```python
from build123d import *

# Parameters (mm, degrees)
BOSS_EXTRUDE1_DEPTH = 20
SHELL4_T            = 2
FILLET2_R           = 5
SKETCH3_W           = 21.5
SKETCH3_H           = 30
BOSS_EXTRUDE2_DEPTH = 20
SKETCH4_W           = 17.5
SKETCH4_H           = 28
CUT_EXTRUDE1_DEPTH  = 3.3
CUT_EXTRUDE2_DEPTH  = 2


with BuildPart() as part:
    # Sketch2 → Boss-Extrude1 (new body)
    with BuildSketch(Plane(origin=(0, 0, 0), x_dir=(0, 0, -1), z_dir=(1, 0, 0))):
        with BuildLine():
            Line((-27.001202387, 32.141013477), (-22.602835252, -36.63027149))
            ThreePointArc((-22.602835252, -36.63027149), (-19.464913087, -43.285247796), (-12.623224858, -45.992011054))
            Line((-12.623224858, -45.992011054), (12.623224858, -45.992011054))
            ThreePointArc((12.623224858, -45.992011054), (19.464913087, -43.285247796), (22.602835252, -36.63027149))
            Line((22.602835252, -36.63027149), (27.001202387, 32.141013477))
            ThreePointArc((27.001202387, 32.141013477), (25.118351891, 38.648045435), (19.520174304, 42.462098214))
            ThreePointArc((19.520174304, 42.462098214), (0, 44.940033366), (-19.520174304, 42.462098214))
            ThreePointArc((-19.520174304, 42.462098214), (-25.118351891, 38.648045435), (-27.001202387, 32.141013477))
        make_face()
    extrude(amount=BOSS_EXTRUDE1_DEPTH)

    # Shell4
    shell4_openings = [part.faces().sort_by_distance(p)[0] for p in [
        (20, 0.52350314, 0),
    ]]
    offset(amount=SHELL4_T, openings=shell4_openings, kind=Kind.INTERSECTION)

    # Fillet2
    # the kernel refuses this fillet: 5 mm, written as the material it takes off along each edge
    with BuildSketch(Plane(origin=(-2, -47.992011054, 12.623224858), x_dir=(1, 0, 0), z_dir=(0, 0, -1))) as fillet2_piece_1:
        with BuildLine():
            CenterArc((FILLET2_R, -FILLET2_R), FILLET2_R, 90, 90)
            Line((0, -FILLET2_R), (0, 0))
            Line((0, 0), (FILLET2_R, 0))
        make_face()
    extrude(amount=25.246449717, mode=Mode.SUBTRACT)
    with BuildSketch(Plane(origin=(-2, -35.992011054, 12.623224858), x_dir=(0, -1, 0), z_dir=(0, 0, -1))) as fillet2_piece_2:
        with BuildLine():
            CenterArc((12 - FILLET2_R, -FILLET2_R), FILLET2_R, 0, 90)
            Line((12 - FILLET2_R, 0), (12, 0))
            Line((12, 0), (12, -FILLET2_R))
        make_face()
    revolve(axis=Axis((-2, -35.992011054, 12.623224858), (-1, 0, 0)), revolution_arc=86.340549578, mode=Mode.SUBTRACT)
    with BuildSketch(Plane(origin=(-2, 32.01336139, 28.997124466), x_dir=(1, 0, 0), z_dir=(0, -0.997961039394411, -0.06382604367205215)), Plane(origin=(-2, -36.757923578, -24.598757331), x_dir=(1, 0, 0), z_dir=(0, 0.9979610393944109, -0.06382604367205376))) as fillet2_piece_3:
        with BuildLine():
            CenterArc((FILLET2_R, -FILLET2_R), FILLET2_R, 90, 90)
            Line((0, -FILLET2_R), (0, 0))
            Line((0, 0), (FILLET2_R, 0))
        make_face()
    extrude(amount=68.911793399, mode=Mode.SUBTRACT)
    with BuildSketch(Plane(origin=(-2, 32.779273914, 17.021591993), x_dir=(0, -0.06382604367205197, 0.997961039394411), z_dir=(0, -0.997961039394411, -0.06382604367205197))) as fillet2_piece_4:
        with BuildLine():
            CenterArc((12 - FILLET2_R, -FILLET2_R), FILLET2_R, 0, 90)
            Line((12 - FILLET2_R, 0), (12, 0))
            Line((12, 0), (12, -FILLET2_R))
        make_face()
    revolve(axis=Axis((-2, 32.779273914, 17.021591993), (-1, 0, 0)), revolution_arc=79.190327228, mode=Mode.SUBTRACT)
    with BuildSketch(Plane(origin=(-2, -33.184966634, 0), x_dir=(0, 0.9682824300555203, 0.249858231094708), z_dir=(0, -0.249858231094708, 0.9682824300555203))) as fillet2_piece_5:
        with BuildLine():
            CenterArc((80.125 - FILLET2_R, -FILLET2_R), FILLET2_R, 0, 90)
            Line((80.125 - FILLET2_R, 0), (80.125, 0))
            Line((80.125, 0), (80.125, -FILLET2_R))
        make_face()
    revolve(axis=Axis((-2, -33.184966634, 0), (-1, 0, 0)), revolution_arc=28.938246388, mode=Mode.SUBTRACT)
    with BuildSketch(Plane(origin=(-2, 32.779273914, -17.021591993), x_dir=(0, 0.9682824300555204, -0.24985823109470737), z_dir=(0, 0.24985823109470737, 0.9682824300555204))) as fillet2_piece_6:
        with BuildLine():
            CenterArc((12 - FILLET2_R, -FILLET2_R), FILLET2_R, 0, 90)
            Line((12 - FILLET2_R, 0), (12, 0))
            Line((12, 0), (12, -FILLET2_R))
        make_face()
    revolve(axis=Axis((-2, 32.779273914, -17.021591993), (-1, 0, 0)), revolution_arc=79.190327228, mode=Mode.SUBTRACT)
    with BuildSketch(Plane(origin=(-2, -35.992011054, -12.623224858), x_dir=(0, -0.06382604367205372, -0.9979610393944109), z_dir=(0, 0.9979610393944109, -0.06382604367205372))) as fillet2_piece_7:
        with BuildLine():
            CenterArc((12 - FILLET2_R, -FILLET2_R), FILLET2_R, 0, 90)
            Line((12 - FILLET2_R, 0), (12, 0))
            Line((12, 0), (12, -FILLET2_R))
        make_face()
    revolve(axis=Axis((-2, -35.992011054, -12.623224858), (-1, 0, 0)), revolution_arc=86.340549578, mode=Mode.SUBTRACT)

    # Sketch3 → Boss-Extrude2 (add)
    with BuildSketch(Plane(origin=(0, 0, 0), x_dir=(0, 0, -1), z_dir=(1, 0, 0))):
        with Locations((0, -30.992011054)):
            Rectangle(SKETCH3_W, SKETCH3_H)
    extrude(amount=BOSS_EXTRUDE2_DEPTH)

    # Sketch4 → Cut-Extrude1 (cut)
    with BuildSketch(Plane(origin=(20, 0, 0), x_dir=(0, 0, -1), z_dir=(1, 0, 0))):
        with Locations((0, -31.992011054)):
            Rectangle(SKETCH4_W, SKETCH4_H)
    extrude(amount=-CUT_EXTRUDE1_DEPTH, mode=Mode.SUBTRACT)

    # Sketch5 → Cut-Extrude2 (cut)
    with BuildSketch(Plane.XZ.offset(47.992011054)):
        with BuildLine():
            Line((20, 2.351775142), (20, -6.648224858))
            ThreePointArc((20, -6.648224858), (18.961461825, -6.347856856), (18.3, -5.492724858))
            Line((18.3, -5.492724858), (18.3, 1.197275142))
            ThreePointArc((18.3, 1.197275142), (18.954546218, 2.062330624), (20, 2.351775142))
        make_face()
    extrude(amount=-CUT_EXTRUDE2_DEPTH, mode=Mode.SUBTRACT)


solid = part.part
```
Source: CAD feature listing. Evaluate the final solid. Frame: model axes, mm. A direction names the side the tool comes from. Coordinates: 2 decimals unless noted, no trailing zeros. Write each loop counter-clockwise with the first axis right and the second up, starting at its lowest first coordinate (ties: lowest second). Pieces come first, ordered by that corner, then holes. Notation, with made-up numbers: M -10.5,-11 L 28.5,-11 A10 ccw 28.5,-3 Z; hole C 89,12 d4. An arc over 180 degrees is marked long. Answer as a JSON object with one key per item and string values.
1. Access query for faces 1 (the cylindrical face through (-0.496, -46.566, 0.177)), 2 (the flat face through (18.3, -47, -2)), 3 (the flat face through (18, -32, -8.75)). Directions: +Z, -Z, +X, -X, +Y, -Y. A direction counts if a zero-diameter tool reaches every point of the face in a straight line with its end or side. Return the directions, or none.
Evaluation:
{"face 1": "+Z, -Z, -X, -Y", "face 2": "+X, -Y", "face 3": "+X"}
2. Draft query along Y for faces 4 (the flat face through (-2, 0, 0)), 5 (the flat face through (11.38, -1.89, 26.83)), 6 (the cylindrical face through (9.86, -43.213, 19.541)). Return one class per face: released by +Y, released by -Y, zero draft, split by the parting line, or undercut.
Evaluation:
{"face 4": "zero draft", "face 5": "released by -Y", "face 6": "undercut"}
3. Contact query for flat-ended pins moving along their axis: P1, Ø1.5, axis at x = 14, y = 28.5, coming from the +Z side; P2, Ø6, axis at x = 10, y = -25.5, coming from the +Z side; P3, Ø1, axis at x = 19, y = -32, coming from the +Z side. Output: stop coordinate, or through.
Evaluation:
{"P1": "z = 28.82", "P2": "z = 25.51", "P3": "z = 24.94"}
4. Cut plane A-A on x = 7.5. Output: boundary loops of the cut face in (y, z) (3 decimals), plus the area to 3 significant figures.
Evaluation:
{"outline": "M -47.992,-12.623 A12 ccw -36.758,-24.599 L 32.013,-28.997 A12 ccw 44.399,-20.02 A80.125 ccw 44.399,20.02 A12 ccw 32.013,28.997 L -36.758,24.599 A12 ccw -47.992,12.623 Z; hole M -45.992,-12.623 A10 ccw -36.63,-22.603 L 32.141,-27.001 A10 ccw 42.462,-19.52 A78.125 ccw 42.462,19.52 A10 ccw 32.141,27.001 L -36.63,22.603 A10 ccw -45.992,12.623 L -45.992,10.75 L -15.992,10.75 L -15.992,-10.75 L -45.992,-10.75 Z", "area": "1,180 mm^2"}
5. Ray query, L1, parallel to Y at x = 18.25, z = 5; L2, parallel to Z at x = 4.75, y = -19.5; L3, parallel to X at y = 30, z = -6. Return the intervals inside material, ascending.
Evaluation:
{"L1": "-47.99 to -45.99, -17.99 to -15.99, 44.78 to 46.78", "L2": "-25.7 to -23.7, -10.75 to 10.75, 23.7 to 25.7", "L3": "-2 to 0"}
6. Cut plane B-B on x = 2. Output: boundary loops of the cut face in (y, z) (3 decimals), plus the area to 3 significant figures.
Evaluation:
{"outline": "M -47.891,-12.623 A11.899 ccw -36.751,-24.498 L 32.02,-28.896 A11.899 ccw 44.301,-19.995 A80.024 ccw 44.301,19.995 A11.899 ccw 32.02,28.896 L -36.751,24.498 A11.899 ccw -47.891,12.623 Z; hole M -45.992,-12.623 A10 ccw -36.63,-22.603 L 32.141,-27.001 A10 ccw 42.462,-19.52 A78.125 ccw 42.462,19.52 A10 ccw 32.141,27.001 L -36.63,22.603 A10 ccw -45.992,12.623 L -45.992,10.75 L -15.992,10.75 L -15.992,-10.75 L -45.992,-10.75 Z", "area": "1,150 mm^2"}
